from build123d import *


with BuildPart() as f3:
    # F3: sweep along a path in F0
    with BuildLine(Plane.XY) as f3_path:
        Line((-49.0501374006, 27.5603476912), (-49.0501374006, -36.0591337085))
        Line((-49.0501374006, -36.0591337085), (54.1494078934, -36.0591337085))
        Line((54.1494078934, -36.0591337085), (54.1494078934, 27.5603476912))
        Line((54.1494078934, 27.5603476912), (-49.0501374006, 27.5603476912))
    # F2 (on line) → F3 (sweep)
    with BuildSketch(Plane.XZ.offset(36.0591337085)):
        with BuildLine():
            Line((-41.6731166029, 5.010060966), (-57.0862477338, 5.010060966))
            ThreePointArc((-57.0862477338, 5.010060966), (-58.882298958, 4.2661121902), (-59.6262477338, 2.470060966))
            Line((-59.6262477338, 2.470060966), (-59.6262477338, -1.477370753))
            ThreePointArc((-59.6262477338, -1.477370753), (-58.882298958, -3.2734219772), (-57.0862477338, -4.017370753))
            Line((-57.0862477338, -4.017370753), (-41.6731166029, -4.017370753))
            ThreePointArc((-41.6731166029, -4.017370753), (-39.8770653787, -3.2734219772), (-39.1331166029, -1.477370753))
            Line((-39.1331166029, -1.477370753), (-39.1331166029, 2.470060966))
            ThreePointArc((-39.1331166029, 2.470060966), (-39.8770653787, 4.2661121902), (-41.6731166029, 5.010060966))
        make_face()
    sweep(path=f3_path.line, transition=Transition.RIGHT)


solid = f3.part
Geometry: final body of the model. Coordinates: model frame, mm. A direction names the side the tool comes from. Round coordinates to 2 decimals unless told otherwise and drop trailing zeros. Loops run counter-clockwise (first coordinate to the right, second up) from the corner with the lowest first, then second, coordinate; pieces in that order, holes last.
Q1. Section C-C on z = 0.25. Return loops of the section in (x, y), plus the area to 3 significant figures.
Q2. Material intervals for L1, parallel to Y at x = 43.5, z = -0.25; L2, parallel to X at y = 5, z = 0.75; L3, parallel to Y at x = -6.5, z = 2.75, sorted ascending.
Q3. Section A-A on y = -7. Return loops of the section in (x, z).
Q4. Pin query (flat end, axial travel): P1, Ø4, axis at x = -25, y = -24.5, coming from the -Z side. Return the tip coordinate at first contact, or that it passes through.
Q5. Pull-direction query (X, two-part tool) for faces 4 (the flat face through (64.726, -4, 1)), 5 (the cylindrical face through (3.17, -26.87, 4.25)), 6 (the flat face through (3, -31, 5.01)), 7 (the cylindrical face through (-58.902, -4.843, -3.254)); classes: released by +X, released by -X, zero draft, split by the parting line, or undercut.
Q6. Section B-B on x = 32. Return loops of the section in (y, z), plus the area to 3 significant figures.
Q7. Section D-D on x = 45.5. Return loops of the section in (y, z).
Q8. Access query for faces 1 (the flat face through (3, -26.142, 0)), 2 (the cylindrical face through (44.96, -3.91, 4.25)), 3 (the cylindrical face through (44.996, -3.907, -3.293)). Directions: +Z, -Z, +X, -X, +Y, -Y. A direction counts if a zero-diameter tool reaches every point of the face in a straight line with its end or side. Return the directions, or none.
Evaluation:
1. outline: (-59.63, -46.64) - (64.73, -46.64) - (64.73, 38.14) - (-59.63, 38.14) - close; hole (-39.13, -26.14) - (44.23, -26.14) - (44.23, 17.64) - (-39.13, 17.64) - close
1. area: 6,890 mm2
2. L1: y = -46.64 to -26.14, 17.64 to 38.14
2. L2: x = -59.63 to -39.13, 44.23 to 64.73
2. L3: y = -46.62 to -26.16, 17.66 to 38.12
3. outline: (-59.63, -1.48) arc R2.54 ccw to (-57.09, -4.02) - (-41.67, -4.02) arc R2.54 ccw to (-39.13, -1.48) - (-39.13, 2.47) arc R2.54 ccw to (-41.67, 5.01) - (-57.09, 5.01) arc R2.54 ccw to (-59.63, 2.47) - close; (44.23, -1.48) arc R2.54 ccw to (46.77, -4.02) - (62.19, -4.02) arc R2.54 ccw to (64.73, -1.48) - (64.73, 2.47) arc R2.54 ccw to (62.19, 5.01) - (46.77, 5.01) arc R2.54 ccw to (44.23, 2.47) - close
4. P1: stops at z = -2.78
5. face 4: released by +X
5. face 5: undercut
5. face 6: zero draft
5. face 7: released by -X
6. outline: (-46.64, -1.48) arc R2.54 ccw to (-44.1, -4.02) - (-28.68, -4.02) arc R2.54 ccw to (-26.14, -1.48) - (-26.14, 2.47) arc R2.54 ccw to (-28.68, 5.01) - (-44.1, 5.01) arc R2.54 ccw to (-46.64, 2.47) - close; (17.64, -1.48) arc R2.54 ccw to (20.18, -4.02) - (35.6, -4.02) arc R2.54 ccw to (38.14, -1.48) - (38.14, 2.47) arc R2.54 ccw to (35.6, 5.01) - (20.18, 5.01) arc R2.54 ccw to (17.64, 2.47) - close
6. area: 359 mm2
7. outline: (-46.64, -1.48) arc R2.54 ccw to (-44.1, -4.02) - (-28.68, -4.02) arc R2.54 ccw to (-27.41, -3.68) - (18.91, -3.68) arc R2.54 ccw to (20.18, -4.02) - (35.6, -4.02) arc R2.54 ccw to (38.14, -1.48) - (38.14, 2.47) arc R2.54 ccw to (35.6, 5.01) - (20.18, 5.01) arc R2.54 ccw to (18.91, 4.67) - (-27.41, 4.67) arc R2.54 ccw to (-28.68, 5.01) - (-44.1, 5.01) arc R2.54 ccw to (-46.64, 2.47) - close
8. face 1: +Z, -Z
8. face 2: +Z
8. face 3: -Z
